Model file for the job. Use its own axes, mm. A direction names the side the tool comes from. Round coordinates to 2 decimals unless told otherwise and drop trailing zeros. Loops run counter-clockwise (first coordinate to the right, second up) from the corner with the lowest first, then second, coordinate; pieces in that order, holes last. Notation, with made-up numbers: M -23.5,85.25 L 22.5,85.25 A19 cw 22.5,103.25 Z; hole C 83,50 d2. An arc over 180 degrees is marked long. Use a Markdown table: item, result. Add a question column.
Q1. Tool access for faces 1 (the face through (2.8, -0.1, 18.1)), 2 (the face through (-22.15, -9.24, 7.54)): list every direction of +Z, -Z, +X, -X, +Y, -Y with a clear straight run to the whole face (end or side of a thin tool).
Q2. Cut at B-B (z = 27). Give the cut face in (x, y).
Q3. Probe line 1 (Y direction, x = 0, z = 20.25); line 2 (Z direction, x = -6, y = 14); line 3 (Y direction, x = 10, z = 25.5). List the from-to ranges inside material, lowest first. Write a range as from..to.
Q4. Pin check, flat tips, straight feed: pin 1 (14 mm diameter, centred on x = 7, y = 8.5, fed in from +Z); pin 2 (1 mm diameter, centred on x = 1, z = 8.5, fed in from +Y); pin 3 (4 mm diameter, centred on x = 16, y = 1, fed in from +Z); pin 4 (6 mm diameter, centred on x = 0.5, y = 0.5, fed in from +Z). Stop position of each tip, or through.
Q5. Mould opens along Y. For faces 3 (the face through (0.154, 0.695, 1.788)), 4 (the face through (0.103, -18.973, 6.041)), 5 (the face through (13.34, 13.49, 6.04)), 6 (the face through (9.128, 22.197, 7.535)) say: +Y half, -Y half, draft (parallel to the pull), parting line (faces both ways), or undercut.
Q6. Cut at A-A (z = 9). Give the cut face in (x, y), plus the area to 3 significant figures.
from build123d import *

# Parameters (mm, degrees)
SCHNITT_LINEAR_AUSTRAGEN1_DEPTH = 35
KREISMUSTER1_COUNT              = 8
SKIZZE3_W                       = 2.8
SKIZZE3_H                       = 29.5
FASE1_SIZE                      = 2


with BuildPart() as part:
    # Skizze1 → Rotation1 (revolve)
    with BuildSketch(Plane(origin=(0, 0, 0), x_dir=(1, 0, 0), z_dir=(0, 1, 0))):
        Polygon((0, 0), (-19, 0), (-24, -5), (-24, -10), (-12.5, -10), (-12.5, -34), (0, -34), align=None)
    revolve(axis=Axis((0, 0, 34), (0, 0, -1)))

    # Skizze2 → Schnitt-Linear austragen1 (cut, through all)
    with BuildSketch(Plane.XY):
        with BuildLine():
            ThreePointArc((-5, 23.473389189), (0, 18.972344588), (5, 23.473389189))
            ThreePointArc((5, 23.473389189), (0, 24), (-5, 23.473389189))
        make_face()
    schnitt_linear_austragen1 = extrude(amount=SCHNITT_LINEAR_AUSTRAGEN1_DEPTH, mode=Mode.SUBTRACT)

    # Kreismuster1: Schnitt-Linear austragen1 ×8 about axis
    kreismuster1_axis = Axis((0, 0, 0), (0, 0, 1))
    for i in range(1, KREISMUSTER1_COUNT):
        add(schnitt_linear_austragen1.rotate(kreismuster1_axis, i * 360 / KREISMUSTER1_COUNT), mode=Mode.SUBTRACT)

    # Skizze3 → Schnitt-Rotation1 (revolve, cut)
    with BuildSketch(Plane(origin=(0, 0, 0), x_dir=(1, 0, 0), z_dir=(0, 1, 0))):
        Polygon((0, 0), (0, -2.5), (-2.5, 0), align=None)
        with Locations((-1.4, -19.25)):
            Rectangle(SKIZZE3_W, SKIZZE3_H)
    revolve(axis=Axis((0, 0, 0), (0, 0, 1)), mode=Mode.SUBTRACT)

    # Fase1
    fase1_edges = [part.edges().sort_by_distance(p)[0] for p in [
        (2.8, 0, 34),
        (12.5, 0, 34),
    ]]
    chamfer(fase1_edges, length=FASE1_SIZE)


solid = part.part
Checked values:
| question | item | result |
|---|---|---|
| 1 | face 1 | +Z |
| 1 | face 2 | +Z, -Z, -X, -Y |
| 2 | outline | C 0,0 d25; hole C 0,0 d5.6 |
| 3 | line 1 | y = -12.5..-2.8, 2.8..12.5 |
| 3 | line 2 | z = 0..10 |
| 3 | line 3 | y = -7.5..7.5 |
| 4 | pin 1 | stops at z = 34 |
| 4 | pin 2 | stops at y = 19.2 |
| 4 | pin 3 | stops at z = 10 |
| 4 | pin 4 | stops at z = 32.91 |
| 5 | face 3 | undercut |
| 5 | face 4 | -Y half |
| 5 | face 5 | undercut |
| 5 | face 6 | +Y half |
| 6 | outline | M -23.47,-5 A24 ccw -20.13,-13.06 A5.03 cw -13.06,-20.13 A24 ccw -5,-23.47 A5.03 cw 5,-23.47 A24 ccw 13.06,-20.13 A5.03 cw 20.13,-13.06 A24 ccw 23.47,-5 A5.03 cw 23.47,5 A24 ccw 20.13,13.06 A5.03 cw 13.06,20.13 A24 ccw 5,23.47 A5.03 cw -5,23.47 A24 ccw -13.06,20.13 A5.03 cw -20.13,13.06 A24 ccw -23.47,5 A5.03 cw Z; hole C 0,0 d5.6 |
| 6 | area | 1,480 mm^2 |
